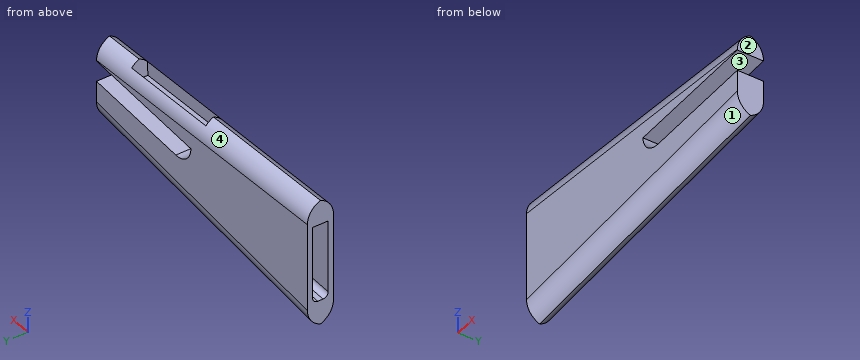
from build123d import *

# Parameters (mm, degrees)
F1_DEPTH    = 6.35
F2_W        = 3.81
F2_H        = 19.05
F3_DEPTH    = 7.62
F4_R        = 1.27
F5_R        = 1.27
F7_DEPTH    = 5.08
F8_T1_DEPTH = 99.3332002554
F8_T3_DEPTH = 99.2137995652
F9_R        = 5.07999


# Not quite as in the source:
# - a fillet or chamfer that OpenCascade refuses, or shapes differently, is made with other operations: its cross-section is extruded or revolved along the edge and cut away or added
# - a fillet or chamfer is up to 0.001 mm smaller than in the source, because OpenCascade refuses the exact size


with BuildPart() as f1:
    # F0 (on Front) → F1 (new body)
    with BuildSketch(Plane.XZ):
        Polygon((28.8813739334, 7.6191808492), (28.8813739334, 12.8777329371), (-44.7786260666, 17.6402329371), (-44.7786260666, -14.1097670629), (28.8813739334, -7.7597670629), (28.8813739334, 2.5343412086), (-3.8856118554, 1.1037037128), (-4.1071983432, 6.1788686784), align=None)
    extrude(amount=F1_DEPTH)

    # F2 (on face) → F3 (cut)
    with BuildSketch(Plane(origin=(-44.7786260666, 0, 0), x_dir=(0, -1, 0), z_dir=(-1, 0, 0))):
        with Locations((3.175, 1.7652329371)):
            Rectangle(F2_W, F2_H)
    extrude(amount=-F3_DEPTH, mode=Mode.SUBTRACT)

    # F4
    f4_edges = [f1.edges().sort_by_distance(p)[0] for p in [
        (-37.158626, -3.175, -7.759767),
    ]]
    fillet(f4_edges, radius=F4_R)

    # F5
    f5_edges = [f1.edges().sort_by_distance(p)[0] for p in [
        (-37.158626, -3.175, 11.290233),
        (-37.158626, -5.08, 2.400233),
        (-37.158626, -1.27, 2.400233),
    ]]
    fillet(f5_edges, radius=F5_R)

    # F6 (on face) → F7 (cut)
    with BuildSketch(Plane(origin=(0.9493759321, 0, 14.6836810837), x_dir=(0.9979163847, 0, -0.0645204559), z_dir=(0.0645204559, 0, 0.9979163847))):
        Polygon((15.2903190595, -1.27), (2.5903190595, -1.27), (-8.3756055683, -1.27), (-8.3756055683, -5.08), (15.2903190595, -5.08), (17.6343005151, -5.08), (17.6343005151, -1.27), align=None)
    extrude(amount=-F7_DEPTH, mode=Mode.SUBTRACT)

    # F8: fillet of radius 5.08 on 4 edges, made by hand

    # F8_s2 → F8_t1 (cut)
    with BuildSketch(Plane(origin=(-58.308759718, 0, -5.0266172171), x_dir=(0, 1, 0), z_dir=(0.996304769, 0, 0.0858883422))):
        with BuildLine():
            ThreePointArc((-6.35, -5.1316662572), (-4.8621024484, -8.7237687056), (-1.27, -10.2116662572))
            Line((-1.27, -10.2116662572), (-6.35, -10.2116662572))
            Line((-6.35, -10.2116662572), (-6.35, -5.1316662572))
        make_face()
        with BuildLine():
            ThreePointArc((0, -5.1316662572), (-1.4878975516, -8.7237687056), (-5.08, -10.2116662572))
            Line((-5.08, -10.2116662572), (0, -10.2116662572))
            Line((0, -10.2116662572), (0, -5.1316662572))
        make_face()
    extrude(amount=F8_T1_DEPTH, mode=Mode.SUBTRACT)

    # F8_s4 → F8_t3 (cut)
    with BuildSketch(Plane(origin=(40.6055360865, 0, -2.6253579366), x_dir=(0, 1, 0), z_dir=(-0.9979163847, 0, 0.0645204559))):
        with BuildLine():
            ThreePointArc((-1.27, -14.7143401085), (-4.8621024484, -13.2264425569), (-6.35, -9.6343401085))
            Line((-6.35, -9.6343401085), (-6.35, -14.7143401085))
            Line((-6.35, -14.7143401085), (-1.27, -14.7143401085))
        make_face()
        with BuildLine():
            ThreePointArc((-5.08, -14.7143401085), (-1.4878975516, -13.2264425569), (0, -9.6343401085))
            Line((0, -9.6343401085), (0, -14.7143401085))
            Line((0, -14.7143401085), (-5.08, -14.7143401085))
        make_face()
    extrude(amount=F8_T3_DEPTH, mode=Mode.SUBTRACT)

    # F9 (radius 5.08 in the source; OpenCascade refuses exactly that, so slightly less here)
    f9_edges = [f1.edges().sort_by_distance(p)[0] for p in [
        (-3.885612, -3.175, 1.103704),
    ]]
    fillet(f9_edges, radius=F9_R)


solid = f1.part
Could you check a few things on this model? Use its own coordinates, in mm. Face numbers are marked on the shaded views. Coordinates: 2 decimals unless noted, no trailing zeros. Answer in a Markdown table with one row per item.
(1) If I drill on probe 1 along X at (y, z) = (-3.25, -5); probe 2 along Y at (x, z) = (-4, 13); probe 3 along Z at (x, y) = (23.5, -2.5), over which ranges is the centre line in solid material (lowest first)?
Results found:
| item | result |
|---|---|
| probe 1 | x = -37.16 to 28.88 |
| probe 2 | y = -5.31 to -5.08, -1.27 to -1.04 |
| probe 3 | z = -7.52 to 2.3, 7.38 to 12.52 |
(2) Thinking about a two-plate mould opening in Z: for the marked faces 1, 2, 3 and 4, which applies, released by +Z, released by -Z, zero draft, split by the parting line, or undercut?
Results found:
| item | result |
|---|---|
| face 1 | released by -Z |
| face 2 | zero draft |
| face 3 | undercut |
| face 4 | released by +Z |
(3) Will these pins go through, and if not, where does the flat tip stop? pin 1 Ø1 at (x, y) = (-42.5, -3) entering from +Z; pin 2 Ø5.5 at (x, z) = (4.5, 11.5) entering from +Y; pin 3 Ø5 at (x, z) = (1, 14) entering from -Y; pin 4 Ø3 at (x, y) = (-5.5, -1.5) entering from -Z.
Results found:
| item | result |
|---|---|
| pin 1 | stops at z = 17.15 |
| pin 2 | stops at y = 0 |
| pin 3 | stops at y = -5.98 |
| pin 4 | stops at z = -10.29 |
